Model file for the job. Use its own axes, mm. Face numbers are marked on the shaded views. A direction names the side the tool comes from. Round coordinates to 2 decimals unless told otherwise and drop trailing zeros. Loops run counter-clockwise (first coordinate to the right, second up) from the corner with the lowest first, then second, coordinate; pieces in that order, holes last. Notation, with made-up numbers: M 46,6 L 81,6 A24 cw 81,28 Z; hole C 43,-27 d2. An arc over 180 degrees is marked long. Use a Markdown table: item, result. Add a question column.
Q1. Pin check, flat tips, straight feed: pin 1 (2 mm diameter, centred on x = -2.5, z = 6, fed in from +Y); pin 2 (6 mm diameter, centred on x = 14.5, y = 2.5, fed in from -Z); pin 3 (1.3 mm diameter, centred on x = 2, z = 2, fed in from +Y). Stop position of each tip, or through.
Q2. Cut at B-B (x = 1.5). Give the cut face in (y, z).
Q3. Cut at C-C (y = -8). Give the cut face in (x, z).
Q4. Probe line 1 (Y direction, x = -19.3, z = 1.8); line 2 (Y direction, x = 19.3, z = 2.05); line 3 (Y direction, x = 20, z = 4.5). List the from-to ranges inside material, lowest first. Write a range as from..to.
Q5. Mould opens along X. For the marked faces 1, 2, 3 and 4 say: +X half, -X half, draft (parallel to the pull), parting line (faces both ways), or undercut.
Q6. Tool access for the marked faces 5 and 6: list every direction of +Z, -Z, +X, -X, +Y, -Y with a clear straight run to the whole face (end or side of a thin tool).
Q7. Cut at A-A (z = 1.75). State how many separate pieces and enclosed holes the cut face has, plus the area to 3 significant figures.
Autodesk Inventor part; units mm, degrees
ref_plane "YZ Plane" through (0, 0, 0) normal (1, 0, 0) x (0, 1, 0)
ref_plane "XZ Plane" through (0, 0, 0) normal (0, 1, 0) x (-1, 0, 0)
ref_plane "XY Plane" through (0, 0, 0) normal (0, 0, 1) x (1, 0, 0)
sketch "Эскиз1" plane through (0, 0, 0) normal (0, 0, 1) x (1, 0, 0)
  arc A0 (-22.3, -16.3) -> (-19.3, -19.3) centre (-19.3, -16.3) ccw
  line L0 (-22.3, -16.3) -> (-22.3, 16.3)
  arc A1 (-19.3, 19.3) -> (-22.3, 16.3) centre (-19.3, 16.3) ccw
  line L1 (-19.3, 19.3) -> (19.3, 19.3)
  arc A2 (22.3, 16.3) -> (19.3, 19.3) centre (19.3, 16.3) ccw
  line L2 (22.3, 16.3) -> (22.3, -16.3)
  arc A3 (19.3, -19.3) -> (22.3, -16.3) centre (19.3, -16.3) ccw
  line L3 (19.3, -19.3) -> (-19.3, -19.3)
  circle A4 centre (19.3, 16.3) radius 2 construction
  circle A5 centre (-19.3, 16.3) radius 2 construction
  circle A6 centre (-19.3, -16.3) radius 2 construction
  circle A7 centre (19.3, -16.3) radius 2 construction
  arc A8 (-1.4869, 14.15) -> (-14.15, 1.4869) centre (-9.15, 9.15) ccw
  line L4 (-14.15, 1.4869) -> (-14.15, -1.4869)
  arc A9 (-14.15, -1.4869) -> (-1.4869, -14.15) centre (-9.15, -9.15) ccw
  line L5 (-1.4869, -14.15) -> (1.4869, -14.15)
  arc A10 (1.4869, -14.15) -> (14.15, -1.4869) centre (9.15, -9.15) ccw
  line L6 (14.15, -1.4869) -> (14.15, 1.4869)
  arc A11 (14.15, 1.4869) -> (1.4869, 14.15) centre (9.15, 9.15) ccw
  line L7 (1.4869, 14.15) -> (-1.4869, 14.15)
  line L8 (-9.15, 9.15) -> (-9.15, 18.3) construction
  line L9 (9.15, 9.15) -> (9.15, 18.3) construction
  line L10 (-9.15, 9.15) -> (-18.3, 9.15) construction
  line L11 (-9.15, -9.15) -> (-18.3, -9.15) construction
  line L12 (-18.3, 9.15) -> (-18.3, -9.15)
  line L13 (-9.15, 18.3) -> (9.15, 18.3)
  line L14 (-22.3, 0) -> (22.3, 0) construction
  line L15 (0, 19.3) -> (0, -19.3) construction
  line L16 (18.3, 9.15) -> (18.3, -9.15)
  line L17 (-9.15, -18.3) -> (9.15, -18.3)
  circle A12 centre (-19.3, 16.3) radius 1.5
  circle A13 centre (19.3, 16.3) radius 1.5
  circle A14 centre (19.3, -16.3) radius 1.5
  circle A15 centre (-19.3, -16.3) radius 1.5
  line L18 (0, 19.3) -> (-7.8, 19.3) construction
  line L19 (-7.8, 19.3) -> (-7.8, 12.8) construction
  line L20 (-7.8, 12.8) -> (0, 12.8) construction
  line L21 (0, 12.8) -> (0, 19.3) construction
  line L22 (-7.8, 12.8) -> (7.8, 12.8)
  line L23 (7.8, 12.8) -> (7.8, 19.3)
  line L24 (7.8, 19.3) -> (-7.8, 19.3)
  line L25 (-7.8, 19.3) -> (-7.8, 12.8)
  line L26 (-18.3, 9.15) -> (-18.3, 4.15) construction
  line L27 (-18.3, -9.15) -> (-18.3, -4.15) construction
  line L28 (-18.3, -4.15) -> (-21.5, -4.15)
  line L29 (-21.5, -4.15) -> (-21.5, 4.15)
  line L30 (-21.5, 4.15) -> (-18.3, 4.15)
  line L31 (-18.3, 4.15) -> (-18.3, -4.15)
  line L32 (18.3, -4.15) -> (21.5, -4.15)
  line L33 (21.5, -4.15) -> (21.5, 4.15)
  line L34 (21.5, 4.15) -> (18.3, 4.15)
  line L35 (18.3, 4.15) -> (18.3, -4.15)
  line L36 (-21.5, 0) -> (-21.5, 12.8)
  line L37 (-21.5, 12.8) -> (-17.5405, 12.8)
  line L38 (-21.5, 0) -> (-21.5, -12.8)
  line L39 (-21.5, -12.8) -> (-17.5405, -12.8)
  point P0 (7.8, 18.1999)
  point P1 (-7.8, 18.1999)
  dimension "d5" = 3
  dimension "d6" = 3
  dimension "d7" = 3
  dimension "d8" = 3
  dimension "d9" = 7.8
  dimension "d10" = 6.5
  dimension "d11" = 15.6
  dimension "d12" = 6.5
  dimension "d13" = 5
  dimension "d14" = 5
  dimension "d15" = 3.2
  dimension "d16" = 8.3
  dimension "d19" = 12.8
extrude "Выдавливание1" add sketch "Эскиз1" along normal blind 6.4 contours L0 A1 L1 L25 L13 A8 L37 L36 L29 L38 L39 A9 L17 A10 L16 L32 L33 L34 A11 L23 A2 L2 A3 L3 A0 | L25 A8 L13 | L13 A11 L23 | A8 L25 L22 L23 A11 L6 A10 L5 A9 L4 | A8 L12 L30 L36 L37 | L16 A10 L6 A11 | A8 L4 A9 L12 | L34 L33 L32 L16 | L12 L28 L29 L30 | L12 A9 L39 L38 L28 | L17 A9 L5 A10
chamfer "Фаска1" distance 2 angle 45 4 edges at (17.8, 16.3, 6.4) (-20.8, 16.3, 6.4) (-20.8, -16.3, 6.4) (17.8, -16.3, 6.4)
extrude "Выдавливание2" cut sketch "Эскиз1" along normal blind 4.4 contours A8 L25 L22 L23 A11 L6 A10 L5 A9 L4 | A8 L12 L30 L36 L37 | L16 A10 L6 A11 | A8 L4 A9 L12 | L34 L33 L32 L16 | L12 L28 L29 L30 | L12 A9 L39 L38 L28 | L17 A9 L5 A10
sketch "Эскиз2" plane through (-22.3, -16.3, 0) normal (-1, 0, 0) x (0, 0, 1)
  line L0 (0, -3) -> (0, 0)
  line L1 (0, 35.6) -> (5.9, 35.6)
  line L2 (0, -3) -> (0, 35.6) construction
  line L3 (0, 16.3) -> (6.4, 16.3) construction
  line L4 (6.4, 30.7972) -> (6.4, 1.8028)
  line L5 (0, 16.3) -> (1, 16.3) construction
  line L6 (1, 16.3) -> (1, 20.5) construction
  line L7 (1, 20.5) -> (0, 20.5) construction
  line L8 (0, 20.5) -> (0, 16.3) construction
  line L9 (1, 20.5) -> (3.6, 20.5)
  line L10 (3.6, 20.5) -> (3.6, 12.1)
  line L11 (3.6, 12.1) -> (1, 12.1)
  line L12 (1, 12.1) -> (1, 20.5)
  line L13 (1, 20.5) -> (2.3, 20.5) construction
  line L14 (2.3, 20.5) -> (2.3, 19.2) construction
  line L15 (2.3, 19.2) -> (1, 19.2) construction
  line L16 (1, 19.2) -> (1, 20.5) construction
  arc A0 (3.6, 19.2) -> (1, 19.2) centre (2.3, 19.2) ccw
  arc A1 (1, 13.4) -> (3.6, 13.4) centre (2.3, 13.4) ccw
  point P0 (3.6, 13.4)
  point P1 (1, 19.2)
  point P2 (1, 13.4)
  point P3 (2.3, 12.1)
  point P4 (2.3, 20.5)
  dimension "d20" = 1
  dimension "d21" = 4.2
  dimension "d22" = 2.6
  dimension "d23" = 8.4
  dimension "d24" = 1.3
  dimension "d25" = 1.3
extrude "Выдавливание3" cut sketch "Эскиз2" against normal blind 0.8 contours A0 L10 A1 L12
fillet "Сопряжение1" radius 2 1 edges at (21.5, 0, 4.4)
properties part number "akkum_cap_pd"
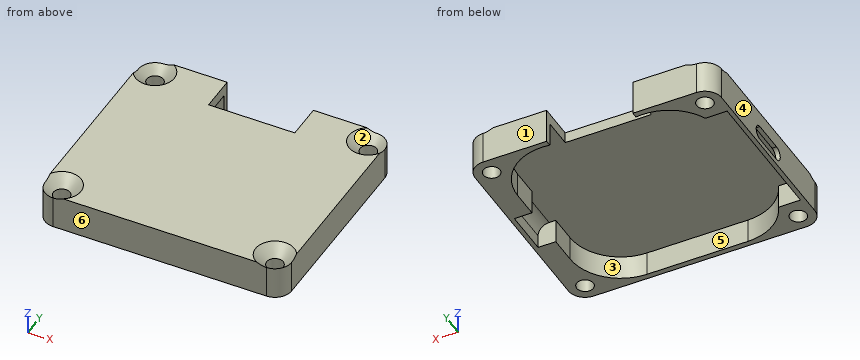
Checked values:
| question | item | result |
|---|---|---|
| 1 | pin 1 | stops at y = 12.8 |
| 1 | pin 2 | stops at z = 4.4 |
| 1 | pin 3 | stops at y = -18.3 |
| 2 | outline | M -19.3,0 L -18.3,0 L -18.3,4.4 L 12.8,4.4 L 12.8,6.4 L -19.3,6.4 Z |
| 3 | outline | M -22.3,0 L -21.5,0 L -21.5,4.4 L 18.3,4.4 L 18.3,0 L 22.3,0 L 22.3,6.4 L -22.3,6.4 Z |
| 4 | line 1 | y = -19.3..-17.8, -14.8..-12.8, 12.8..14.8, 17.8..19.3 |
| 4 | line 2 | y = -19.3..-17.8, -14.8..-4.15, 4.15..14.8, 17.8..19.3 |
| 4 | line 3 | y = -19.22..-17.74, -14.86..14.86, 17.74..19.22 |
| 5 | face 1 | draft |
| 5 | face 2 | undercut |
| 5 | face 3 | undercut |
| 5 | face 4 | -X half |
| 6 | face 5 | -Z |
| 6 | face 6 | +Z, -Z, +X, -X, -Y |
| 7 | separate pieces | 2 |
| 7 | enclosed holes | 4 |
| 7 | area | 286 mm^2 |
